The model under review builds one solid part; all positions refer to its coordinate system, in mm. A direction names the side the tool comes from. Give positions to 0.01 mm unless a question says otherwise; leave off trailing zeros. Loops run counter-clockwise (first coordinate to the right, second up) from the corner with the lowest first, then second, coordinate; pieces in that order, holes last. Notation, with made-up numbers: (0.25, 82.25) -> (59.25, 82.25) arc R19 ccw to (59.25, 99.25) -> close; hole circle Ø9 at (-24.5, 78). An arc over 180 degrees is marked (long way). Write each question's results on one line, items separated by ' | '. Start each with the question number.
Q1. Mouldability with a two-part tool opening along Z and no side actions: class faces 3 (the face through (-3.7, -1.2, -2.3)), 4 (the face through (-0.1, -0.6, 2.5)), 5 (the face through (2.4, 0.3, 4.1)), 6 (the face through (2.342, 0.304, -4.133)) as released by +Z, released by -Z, zero draft, split by the parting line, or undercut.
Q2. Wall thickness on L1, parallel to X at y = 0.1, z = 0; L2, parallel to X at y = -0.05, z = 0; L3, parallel to Y at x = -4, z = -2.75: over which ranges is each line inside the solid? List them lowest first. Write a range as [from, to].
Q3. Insertion check: pin 1 Ø5.5 at (x, z) = (0, 0) entering from +Y. The pin has a flat end and moves straight along its axis. Give the tip position at first contact, or say it passes through.
Q4. We need section B-B (y = -0.6). Write out the cut boundary in (x, z), plus the area to 3 significant figures.
Q5. Machinability: for faces 1 (the face through (3, -1.7, -1)), 2 (the face through (-4, 0, 2)), which of the approach directions +Z, -Z, +X, -X, +Y, -Y give a long, thin tool a straight path to every point of the face, cutting with its end or side? Answer none if there is none.
from build123d import *

# Parameters (mm, degrees)
HEXDIESKE_R  = 5.5105
HEXDIE_DEPTH = 0.6


with BuildPart() as part:
    # BodySke → Body (revolve)
    with BuildSketch(Plane.XY, mode=Mode.PRIVATE) as body_sk:
        Polygon((4.066324865, 0), (5.5095, 0), (5.5095, 0.6), (2.5, 0.6), (2.5, -1.7), (4.355, -1.7), (4.355, -0.8), (4.066324865, -0.3), align=None)
    revolve(body_sk.sketch.rotate(Axis((0, 0, 0), (0, 1, 0)), 90), axis=Axis((0, 0, 0), (0, 1, 0)))

    # EndChamferSke → EndChamfer (revolve, cut)
    with BuildSketch(Plane.XY, mode=Mode.PRIVATE) as endchamfer_sk:
        Polygon((3, -1.954), (3, -1.69746), (2.5, -1.347486267), (2.5, -1.954), align=None)
        Polygon((3, 0.59746), (2.5, 0.247486267), (2.5, 0.854), (3, 0.854), align=None)
    revolve(endchamfer_sk.sketch.rotate(Axis((0, -2.54, 0), (0, 1, 0)), 90), axis=Axis((0, -2.54, 0), (0, 1, 0)), mode=Mode.SUBTRACT)

    # HexDieSke → HexDie (cut)
    with BuildSketch(Plane(origin=(0, 0.6, 0), x_dir=(-1, 0, 0), z_dir=(0, 1, 0))):
        Circle(HEXDIESKE_R)
        Polygon((0, 5.484827557), (4.75, 2.742413779), (4.75, -2.742413779), (0, -5.484827557), (-4.75, -2.742413779), (-4.75, 2.742413779), align=None, mode=Mode.SUBTRACT)
    extrude(amount=-HEXDIE_DEPTH, mode=Mode.SUBTRACT)


solid = part.part
Output:
1) face 3: split by the parting line | face 4: undercut | face 5: released by +Z | face 6: released by -Z
2) L1: [-4.75, -2.5], [2.5, 4.75] | L2: [-4.07, -2.5], [2.5, 4.07] | L3: [0, 0.6]
3) pin 1: y = 0.42
4) outline: circle Ø8.48 at (0, 0); hole circle Ø5 at (0, 0) | area: 36.8 mm2
5) face 1: +Z, -Z, +X, -X, -Y | face 2: none
